Model file for the job. Use its own axes, mm. A direction names the side the tool comes from. Coordinates: 2 decimals unless noted, no trailing zeros. Order: outer loops, then holes, each group sorted by start corner. A loop starts at its lowest first (then second) coordinate and runs counter-clockwise, first axis right, second up.
from build123d import *

# Parameters (mm, degrees)
BOSS_EXTRUDE1_DEPTH = 19.05


with BuildPart() as part:
    # Sketch1 → Boss-Extrude1 (new body)
    with BuildSketch(Plane(origin=(0, 0, 0), x_dir=(1, 0, 0), z_dir=(0, 1, 0))):
        Polygon((68.696644766, 0), (59.493039522, 34.348322383), (34.348322383, 59.493039522), (0, 68.696644766), (-34.348322383, 59.493039522), (-59.493039522, 34.348322383), (-68.696644766, 0), (-59.493039522, -34.348322383), (-34.348322383, -59.493039522), (0, -68.696644766), (34.348322383, -59.493039522), (59.493039522, -34.348322383), align=None)
        Polygon((25.308220045, 0), (21.917561483, 12.654110022), (12.654110022, 21.917561483), (0, 25.308220045), (-12.654110022, 21.917561483), (-21.917561483, 12.654110022), (-25.308220045, 0), (-21.917561483, -12.654110022), (-12.654110022, -21.917561483), (0, -25.308220045), (12.654110022, -21.917561483), (21.917561483, -12.654110022), align=None, mode=Mode.SUBTRACT)
    extrude(amount=BOSS_EXTRUDE1_DEPTH)


solid = part.part
Q1. Probe line 1 (Z direction, x = 0, y = 12.75); line 2 (Z direction, x = -12, y = 10.75); line 3 (X direction, y = 14.25, z = -16). List the from-to ranges inside material, lowest first.
Established:
line 1: z = -68.7 to -25.31, 25.31 to 68.7
line 2: z = -65.48 to -22.09, 22.09 to 65.48
line 3: x = -64.41 to -18.57, 18.57 to 64.41
Q2. Cut at A-A, the plane y = 2. List the corners of the cut face in (x, z).
Established:
outline: (-68.7, 0) - (-59.49, -34.35) - (-34.35, -59.49) - (0, -68.7) - (34.35, -59.49) - (59.49, -34.35) - (68.7, 0) - (59.49, 34.35) - (34.35, 59.49) - (0, 68.7) - (-34.35, 59.49) - (-59.49, 34.35) - close; hole (-25.31, 0) - (-21.92, -12.65) - (-12.65, -21.92) - (0, -25.31) - (12.65, -21.92) - (21.92, -12.65) - (25.31, 0) - (21.92, 12.65) - (12.65, 21.92) - (0, 25.31) - (-12.65, 21.92) - (-21.92, 12.65) - close
Q3. Cut at B-B, the plane z = 15. List the corners of the cut face in (x, y).
Established:
outline: (-64.68, 0) - (-19.57, 0) - (-19.57, 19.05) - (-64.68, 19.05) - close; (19.57, 0) - (64.68, 0) - (64.68, 19.05) - (19.57, 19.05) - close
Q4. Drop flat-ended pins along their axis: P1, Ø8, axis at x = 51.5, y = 13.5, coming from the +Z side; P2, Ø5, axis at y = 7.5, z = -16.5, coming from the -X side; P3, Ø3, axis at y = 16.5, z = -18, coming from the -X side. Give the stop position or say it passes through.
Established:
P1: stops at z = 46.34
P2: stops at x = -64.95
P3: stops at x = -64.28
Q5. Mould opens along X. For faces 3 (the face through (-17.22, 9.39, -17.35)), 4 (the face through (30, 0, -1)), 5 (the face through (-64.16, 9.39, 16.93)) say: pulls with the +X half, pulls with the -X half, needs draft (parallel to the pull), parting line crosses it, or undercut.
Established:
face 3: undercut
face 4: needs draft
face 5: pulls with the -X half
Q6. Cut at C-C, the plane z = -8. List the corners of the cut face in (x, y), plus the area to 3 significant figures.
Established:
outline: (-66.55, 0) - (-23.16, 0) - (-23.16, 19.05) - (-66.55, 19.05) - close; (23.16, 0) - (66.55, 0) - (66.55, 19.05) - (23.16, 19.05) - close
area: 1,650 mm2
Q7. Cut at D-D, the plane x = 49. List the corners of the cut face in (y, z).
Established:
outline: (0, -44.84) - (19.05, -44.84) - (19.05, 44.84) - (0, 44.84) - close
Q8. Which spindle directions (+Z, -Z, +X, -X, +Y, -Y) get a long thin tool onto all of the face, cutting with end or side? Do faces 1 (the face through (-6.42, 9.39, 23.59)), 2 (the face through (16.93, 9.39, 64.16)). Say none if no direction does.
Established:
face 1: +Y, -Y
face 2: +Z, +X, +Y, -Y
